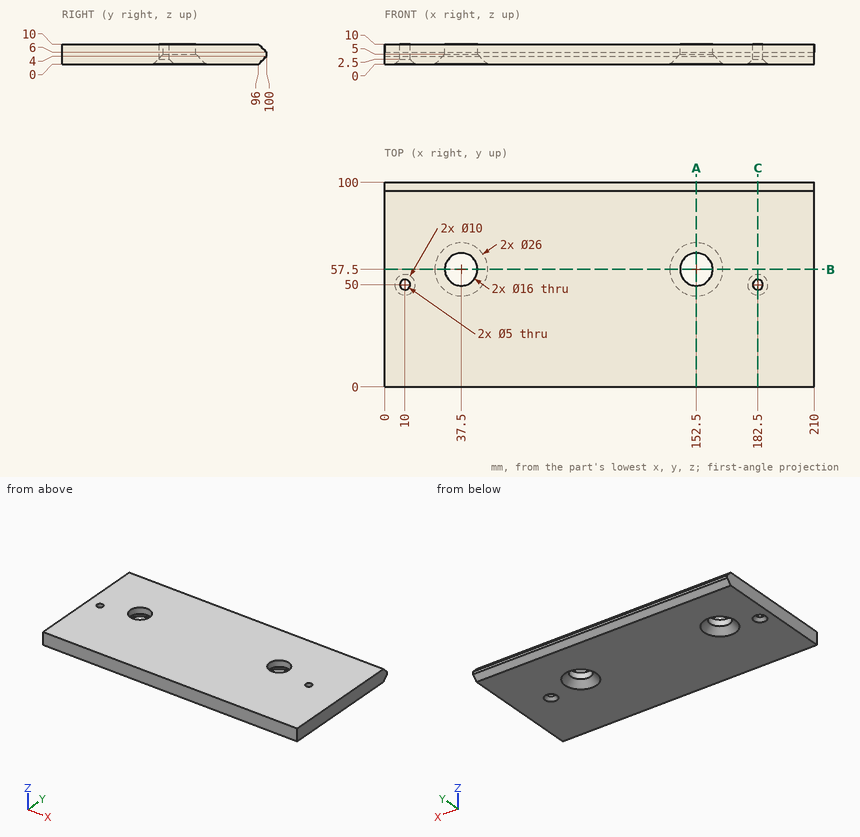
Study the drawing (mm; zero at the part's minimum x, y, z) and answer. Coordinates: 2 decimals unless noted, no trailing zeros. Write each loop counter-clockwise with the first axis right and the second up, starting at its lowest first coordinate (ties: lowest second). Pieces come first, ordered by that corner, then holes. Notation, with made-up numbers: (-11, -1) - (41, -1) arc R25 ccw to (41, 37) - close; hole circle Ø5 at (-12.75, -36). An arc over 180 degrees is marked (long way). Return JSON: item names as keys, results as strings. Group by question number.
1. Straight lines are drawn through the part: L1, parallel to X at y = 57.5, z = 8.7; L2, parallel to Y at x = 181, z = 3.25; L3, parallel to Y at x = 182.5, z = 7.5. For each, find the intervals that lie inside material, in ascending order.
2. Given pin 1 (14.5 mm diameter, centred on x = 152.5, y = 57.5, fed in from -Z), flat-ended and moving along its own axis, determine where the tip first touches the part or whether it passes through.
3. A cutting plane is placed at A-A, the plane x = 152.5. Determine the outline of the cut face in (y, z), plus the area to 3 significant figures.
4. A cutting plane is placed at C-C, the plane x = 182.5. Determine the outline of the cut face in (y, z), plus the area to 3 significant figures.
5. A cutting plane is placed at B-B, the plane y = 57.5. Determine the outline of the cut face in (x, z), plus the area to 3 significant figures.
Ans:
{
 "1": {"L1": "0 to 29.5, 45.5 to 144.5, 160.5 to 210", "L2": "0 to 48, 52 to 99.25", "L3": "0 to 47.5, 52.5 to 98.5"},
 "2": {"pin 1": "through"},
 "3": {"outline": "(0, 0) - (44.5, 0) - (49.5, 5) - (49.5, 10) - (0, 10) - close; (65.5, 5) - (70.5, 0) - (96, 0) - (100, 4) - (100, 6) - (96, 10) - (65.5, 10) - close", "area": "799 mm²"},
 "4": {"outline": "(0, 0) - (45, 0) - (47.5, 2.5) - (47.5, 10) - (0, 10) - close; (52.5, 2.5) - (55, 0) - (96, 0) - (100, 4) - (100, 6) - (96, 10) - (52.5, 10) - close", "area": "928 mm²"},
 "5": {"outline": "(0, 0) - (24.5, 0) - (29.5, 5) - (29.5, 10) - (0, 10) - close; (45.5, 5) - (50.5, 0) - (139.5, 0) - (144.5, 5) - (144.5, 10) - (45.5, 10) - close; (160.5, 5) - (165.5, 0) - (210, 0) - (210, 10) - (160.5, 10) - close", "area": "1,730 mm²"}
}
